from build123d import *

# Parameters (mm, degrees)
F1_DEPTH = 63.5
F2_DEPTH = 25.4
F3_DEPTH = 7.9375
F4_R     = 6.35


with BuildPart() as f1:
    # F0 (on Front) → F1 (new body, symmetric)
    with BuildSketch(Plane.XZ):
        Polygon((-41.275, -9.525), (41.275, -9.525), (41.275, 9.525), (22.225, 9.525), (-41.275, 9.525), align=None)
    extrude(amount=F1_DEPTH, both=True)

    # F0 (on Front) → F2 (join, symmetric)
    with BuildSketch(Plane.XZ):
        with BuildLine():
            Line((22.225, 9.525), (41.275, 9.525))
            Line((41.275, 9.525), (41.275, 27.0002))
            ThreePointArc((41.275, 27.0002), (45.9246798487, 38.2255201513), (57.15, 42.8752))
            Line((57.15, 42.8752), (60.325, 42.8752))
            Line((60.325, 42.8752), (60.325, 61.9252))
            Line((60.325, 61.9252), (57.15, 61.9252))
            add(Edge.make_bspline(
                [(53.8173720822, 61.7658326875), (54.9505591394, 61.8408261866), (56.0622461787, 61.8941638054), (57.15, 61.9252)],
                knots=[108.1113735744, 108.1113735744, 108.1113735744, 108.1113735744, 111.5045361635, 111.5045361635, 111.5045361635, 111.5045361635], degree=3))
            ThreePointArc((53.8173720822, 61.7658326875), (31.3028758367, 50.4881074735), (22.225, 27.0002))
            Line((22.225, 27.0002), (22.225, 9.525))
        make_face()
    extrude(amount=F2_DEPTH, both=True)

    # F0 (on Front) → F3 (join, symmetric)
    with BuildSketch(Plane.XZ):
        with BuildLine():
            add(Edge.make_bspline(
                [(-41.275, 9.525), (-40.218694031, 35.0028870222), (17.7122913335, 59.3764245807), (53.8173720822, 61.7658326875)],
                knots=[0, 0, 0, 0, 108.1113735744, 108.1113735744, 108.1113735744, 108.1113735744], degree=3))
            Line((-41.275, 9.525), (22.225, 9.525))
            Line((22.225, 9.525), (22.225, 27.0002))
            ThreePointArc((22.225, 27.0002), (31.3028758367, 50.4881074735), (53.8173720822, 61.7658326875))
        make_face()
    extrude(amount=F3_DEPTH, both=True)

    # F4
    f4_edges = [f1.edges().sort_by_distance(p)[0] for p in [
        (-41.275, -63.5, 0),
        (41.275, -63.5, 0),
        (41.275, 63.5, 0),
        (-41.275, 63.5, 0),
    ]]
    fillet(f4_edges, radius=F4_R)

    # F0 (on Front) → F5 (revolve)
    with BuildSketch(Plane.XZ):
        Polygon((60.325, 61.9252), (60.325, 42.8752), (85.7551261626, 42.8752), (85.8753103219, 61.9252), align=None)
    revolve(axis=Axis((60.325, 0, 52.3875), (0, 0, 1)))


solid = f1.part
Geometry check sheet. Reference: the model listing, model coordinates, mm. A direction names the side the tool comes from. Give positions to 0.01 mm unless a question says otherwise; leave off trailing zeros. Loops run counter-clockwise (first coordinate to the right, second up) from the corner with the lowest first, then second, coordinate; pieces in that order, holes last. Notation, with made-up numbers: (12, -13.75) -> (18, -13.75) arc R28 ccw to (18, 25.25) -> close; hole circle Ø11 at (-1, 67.25). An arc over 180 degrees is marked (long way). Answer in a Markdown table with one row per item. Add a question column.
1) Cross-section at A-A on z = 1. Record the boundary of the cut face in (x, y) (3 decimals), and give its area (3 significant figures).
2) Set-up check for faces 1 (the face through (22.225, 17, 18)), 2 (the face through (0, -63.5, 0)), 3 (the face through (22.225, -17, 18)), 4 (the face through (41.275, -1, 4)): record each of +Z, -Z, +X, -X, +Y, -Y from which the full face is reachable in a straight line by a thin tool's end or side.
3) Draft check along Z on faces 5 (the face through (36, -25.4, 36)), 6 (the face through (28.014, -16.791, 46.257)), 7 (the face through (34.792, 0.517, 60.012)). Enter one of: pulls with the +Z half, pulls with the -Z half, needs draft (parallel to the pull), parting line crosses it, or undercut.
4) Cross-section at B-B on y = 37. Record the boundary of the cut face in (x, z) (3 decimals), and give its area (3 significant figures).
5) Material ranges on probe 1 along Z at (x, y) = (-24, -11.5) (3 decimals); probe 2 along X at (y, z) = (25, 25.5) (3 decimals); probe 3 along Y at (x, z) = (-11.5, 33.5), recorded low to high. Write a range as from..to.
6) Gauge pin test, flat ends, axial feed: P1, Ø1, axis at x = 47, y = 5, coming from the -Z side; P2, Ø15, axis at x = -18.5, z = 35.5, coming from the +Y side; P3, Ø12, axis at x = 17.5, z = 54.5, coming from the -Y side. Record the tip position at first contact, or that the pin passes through.
Outcome:
| question | item | result |
|---|---|---|
| 1 | outline | (-41.275, -57.15) arc R6.35 ccw to (-34.925, -63.5) -> (34.925, -63.5) arc R6.35 ccw to (41.275, -57.15) -> (41.275, 57.15) arc R6.35 ccw to (34.925, 63.5) -> (-34.925, 63.5) arc R6.35 ccw to (-41.275, 57.15) -> close |
| 1 | area | 10,400 mm^2 |
| 2 | face 1 | +Z, -X, +Y |
| 2 | face 2 | +Z, -Z, +X, -X, -Y |
| 2 | face 3 | +Z, -X, -Y |
| 2 | face 4 | -Z, +X, +Y, -Y |
| 3 | face 5 | needs draft |
| 3 | face 6 | pulls with the +Z half |
| 3 | face 7 | undercut |
| 4 | outline | (-41.275, -9.525) -> (41.275, -9.525) -> (41.275, 9.525) -> (-41.275, 9.525) -> close |
| 4 | area | 1,570 mm^2 |
| 5 | probe 1 | z = -9.525..9.525 |
| 5 | probe 2 | x = 22.225..41.275 |
| 5 | probe 3 | y = -7.94..7.94 |
| 6 | P1 | stops at z = 38.77 |
| 6 | P2 | stops at y = 7.94 |
| 6 | P3 | stops at y = -7.94 |
